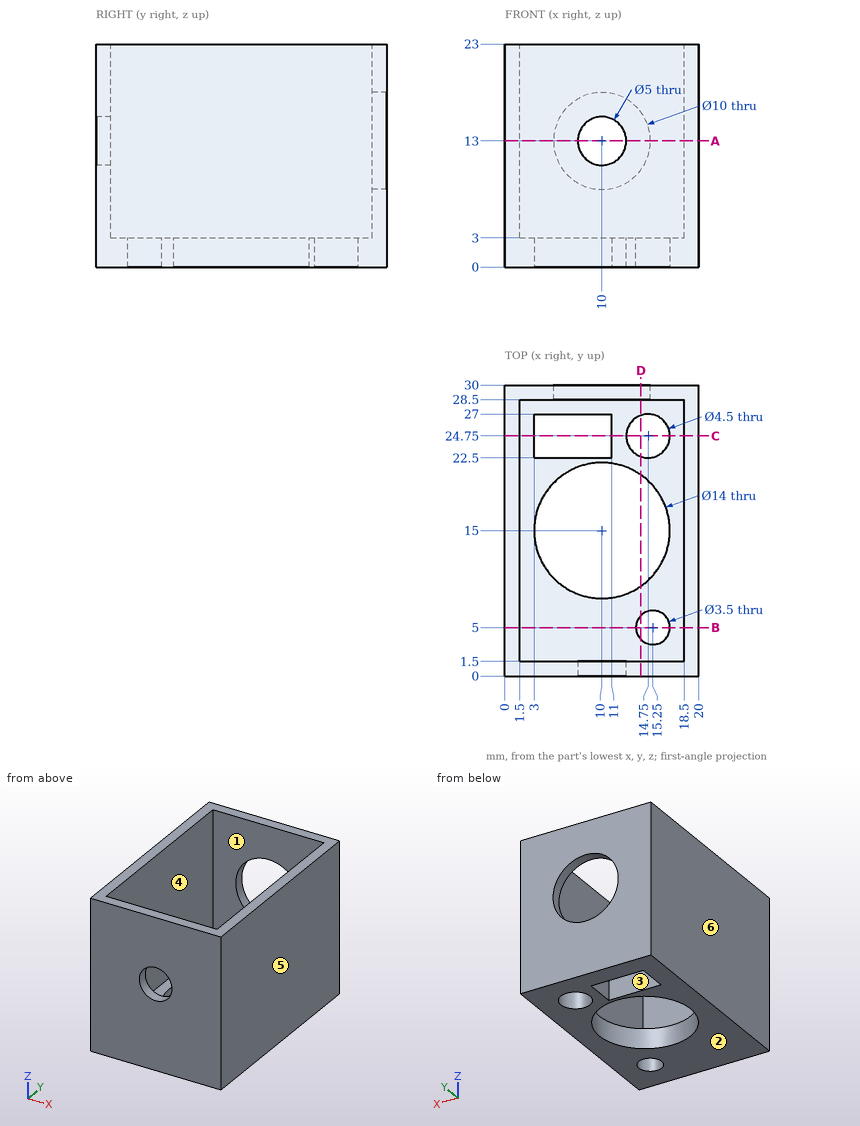
Part print with two shaded views. Sizes in mm from the minimum x, y, z corner. A direction names the side the tool comes from. Round coordinates to 2 decimals unless told otherwise and drop trailing zeros. Order: outer loops, then holes, each group sorted by start corner. A loop starts at its lowest first (then second) coordinate and runs counter-clockwise, first axis right, second up. Notation, with made-up numbers: (-29, -5.5) - (-17, -5.5) arc R24 cw to (-17, 29.5) - close; hole circle Ø2 at (0.5, 75.25). An arc over 180 degrees is marked (long way). Answer in a Markdown table with one row per item. Add a question column.
(1) Mould opens along X. For the marked faces 4, 5 and 6 say: +X half, -X half, draft (parallel to the pull), parting line (faces both ways), or undercut.
(2) 3-axis set-ups, long thin cutter, end or side, ignore diameter. For the marked faces 1, 2 and 3: which of +Z, -Z, +X, -X, +Y, -Y reach the whole face in a straight line?
(3) Drop flat-ended pins along their axis: pin 1 Ø8 at (x, y) = (6, 26.5) entering from -Z; pin 2 Ø6 at (x, y) = (14.75, 24.75) entering from +Z; pin 3 Ø4 at (x, z) = (10, 13) entering from +Y. Give the stop position or say it passes through.
(4) Band-saw the part on C-C on y = 24.75. List the corners of the cut face in (x, z), and give its area (3 significant figures).
(5) Band-saw the part on A-A on z = 13. List the corners of the cut face in (x, y), and give its area (4 significant figures).
(6) Probe L1, parallel to Y at x = 10, z = 1.75; L2, parallel to X at y = 9.75, z = 11.75; L3, parallel to Z at x = 10, y = 0.6. List the from-to ranges inside material, lowest first. Write a range as [from, to].
(7) Band-saw the part on D-D on x = 14. List the corners of the cut face in (y, z).
(8) Band-saw the part on B-B on y = 5. List the corners of the cut face in (x, z).
Data:
| question | item | result |
|---|---|---|
| 1 | face 4 | undercut |
| 1 | face 5 | +X half |
| 1 | face 6 | -X half |
| 2 | face 1 | +Z |
| 2 | face 2 | -Z, +X, -X, +Y, -Y |
| 2 | face 3 | +Z, -Z |
| 3 | pin 1 | stops at z = 0 |
| 3 | pin 2 | stops at z = 3 |
| 3 | pin 3 | passes through |
| 4 | outline | (0, 0) - (3, 0) - (3, 3) - (1.5, 3) - (1.5, 23) - (0, 23) - close; (11, 0) - (12.5, 0) - (12.5, 3) - (11, 3) - close; (17, 0) - (20, 0) - (20, 23) - (18.5, 23) - (18.5, 3) - (17, 3) - close |
| 4 | area | 82.5 mm^2 |
| 5 | outline | (0, 0) - (7.5, 0) - (7.5, 1.5) - (1.5, 1.5) - (1.5, 28.5) - (5, 28.5) - (5, 30) - (0, 30) - close; (12.5, 0) - (20, 0) - (20, 30) - (15, 30) - (15, 28.5) - (18.5, 28.5) - (18.5, 1.5) - (12.5, 1.5) - close |
| 5 | area | 118.5 mm^2 |
| 6 | L1 | y = [0, 8], [22, 22.5], [27, 30] |
| 6 | L2 | x = [0, 1.5], [18.5, 20] |
| 6 | L3 | z = [0, 10.5], [15.5, 23] |
| 7 | outline | (0, 0) - (3.78, 0) - (3.78, 3) - (1.5, 3) - (1.5, 23) - (0, 23) - close; (6.22, 0) - (9.26, 0) - (9.26, 3) - (6.22, 3) - close; (20.74, 0) - (22.63, 0) - (22.63, 3) - (20.74, 3) - close; (26.87, 0) - (30, 0) - (30, 10) - (28.5, 10) - (28.5, 3) - (26.87, 3) - close; (28.5, 16) - (30, 16) - (30, 23) - (28.5, 23) - close |
| 8 | outline | (0, 0) - (13.5, 0) - (13.5, 3) - (1.5, 3) - (1.5, 23) - (0, 23) - close; (17, 0) - (20, 0) - (20, 23) - (18.5, 23) - (18.5, 3) - (17, 3) - close |
